from build123d import *

# Parameters (mm, degrees)
F1_DEPTH = 3


with BuildPart() as f1:
    # F0 (on Front) → F1 (new body)
    with BuildSketch(Plane.XZ):
        with BuildLine():
            Line((11.384419, 13.364318), (16.65998, 18.639879))
            ThreePointArc((16.65998, 18.639879), (9.567086, 23.096988), (1.4, 24.960769))
            Line((1.4, 24.960769), (1.4, 17.5))
            Line((1.4, 17.5), (-1.4, 17.5))
            Line((-1.4, 17.5), (-1.4, 24.960769))
            ThreePointArc((-1.4, 24.960769), (-9.567086, 23.096988), (-16.65998, 18.639879))
            Line((-16.65998, 18.639879), (-11.384419, 13.364318))
            Line((-11.384419, 13.364318), (-13.364318, 11.384419))
            Line((-13.364318, 11.384419), (-18.639879, 16.65998))
            ThreePointArc((-18.639879, 16.65998), (-23.096988, 9.567086), (-24.960769, 1.4))
            Line((-24.960769, 1.4), (-17.5, 1.4))
            Line((-17.5, 1.4), (-17.5, -1.4))
            Line((-17.5, -1.4), (-24.960769, -1.4))
            ThreePointArc((-24.960769, -1.4), (-23.096988, -9.567086), (-18.639879, -16.65998))
            Line((-18.639879, -16.65998), (-13.364318, -11.384419))
            Line((-13.364318, -11.384419), (-11.384419, -13.364318))
            Line((-11.384419, -13.364318), (-16.65998, -18.639879))
            ThreePointArc((-16.65998, -18.639879), (-9.567086, -23.096988), (-1.4, -24.960769))
            Line((-1.4, -24.960769), (-1.4, -17.5))
            Line((-1.4, -17.5), (1.4, -17.5))
            Line((1.4, -17.5), (1.4, -24.960769))
            ThreePointArc((1.4, -24.960769), (9.567086, -23.096988), (16.65998, -18.639879))
            Line((16.65998, -18.639879), (11.384419, -13.364318))
            Line((11.384419, -13.364318), (13.364318, -11.384419))
            Line((13.364318, -11.384419), (18.639879, -16.65998))
            ThreePointArc((18.639879, -16.65998), (23.096988, -9.567086), (24.960769, -1.4))
            Line((24.960769, -1.4), (17.5, -1.4))
            Line((17.5, -1.4), (17.5, 1.4))
            Line((17.5, 1.4), (24.960769, 1.4))
            ThreePointArc((24.960769, 1.4), (23.096988, 9.567086), (18.639879, 16.65998))
            Line((18.639879, 16.65998), (13.364318, 11.384419))
            Line((13.364318, 11.384419), (11.384419, 13.364318))
        make_face()
    extrude(amount=F1_DEPTH)


solid = f1.part
Geometry check sheet. Reference: the model listing, model coordinates, mm. A direction names the side the tool comes from. Give positions to 0.01 mm unless a question says otherwise; leave off trailing zeros. Order: outer loops, then holes, each group sorted by start corner. A loop starts at its lowest first (then second) coordinate and runs counter-clockwise, first axis right, second up. Notation, with made-up numbers: M 40.5,84.25 L 86.5,84.25 A20 ccw 86.5,116.25 Z; hole C -12,26.5 d3. An arc over 180 degrees is marked long. Use a Markdown table: item, result.
Item 1: Tool access check on faces 1 (the flat face through (-17.5, -1, 0)), 2 (the flat face through (-1.4, -1, -21)), 3 (the flat face through (-15.97, -1.48, 13.99)), 4 (the flat face through (21, -1, -1.4)). Record the directions out of +Z, -Z, +X, -X, +Y, -Y that give a thin tool (end or side, any length) a straight path to the whole face; none if there is none.
Answers follow:
| item | result |
|---|---|
| face 1 | -X, +Y, -Y |
| face 2 | -Z, +Y, -Y |
| face 3 | +Y, -Y |
| face 4 | +X, +Y, -Y |
Item 2: Draft check along X on faces 5 (the cylindrical face through (23.05, -1.48, -9.68)), 6 (the flat face through (0, -3, 0)), 7 (the flat face through (16.04, -1.48, 14.06)), 8 (the flat face through (14.06, -1.48, -16.04)). Enter one of: +X half, -X half, draft (parallel to the pull), parting line (faces both ways), or undercut.
Answers follow:
| item | result |
|---|---|
| face 5 | +X half |
| face 6 | draft |
| face 7 | undercut |
| face 8 | undercut |
Item 3: Section check B-B (x = -15). Record the cut outline in (y, z), and give its area (3 significant figures).
Answers follow:
| item | result |
|---|---|
| outline | M -3,-20 L 0,-20 L 0,-16.98 L -3,-16.98 Z; M -3,-13.02 L 0,-13.02 L 0,13.02 L -3,13.02 Z; M -3,16.98 L 0,16.98 L 0,20 L -3,20 Z |
| area | 96.2 mm2 |
Item 4: Material ranges on line 1 along X through (y, z) = (-1.25, 14); line 2 along Z through (x, y) = (-16, -1.7); line 3 along Z through (x, y) = (-15, -2.1), recorded low to high.
Answers follow:
| item | result |
|---|---|
| line 1 | x = -20.71 to -15.98, -12.02 to 12.02, 15.98 to 20.71 |
| line 2 | z = -19.21 to -17.98, -14.02 to 14.02, 17.98 to 19.21 |
| line 3 | z = -20 to -16.98, -13.02 to 13.02, 16.98 to 20 |
Item 5: Section check A-A (z = 15). Record the cut outline in (x, y), and give its area (3 significant figures).
Answers follow:
| item | result |
|---|---|
| outline | M -20,-3 L -16.98,-3 L -16.98,0 L -20,0 Z; M -13.02,-3 L 13.02,-3 L 13.02,0 L -13.02,0 Z; M 16.98,-3 L 20,-3 L 20,0 L 16.98,0 Z |
| area | 96.2 mm2 |
Item 6: Depth check by flat-ended pin: P1, Ø1.5, axis at y = -1, z = 20, coming from the +X side; P2, Ø1.4, axis at x = 0, y = -2, coming from the -Z side; P3, Ø0.8, axis at y = -2, z = -0.5, coming from the +X side. Enter the tip coordinate at first touch or a pass-through.
Answers follow:
| item | result |
|---|---|
| P1 | stops at x = 15.95 |
| P2 | stops at z = -17.5 |
| P3 | stops at x = 17.5 |
Item 7: Section check D-D (x = 20.5). Record the cut outline in (y, z).
Answers follow:
| item | result |
|---|---|
| outline | M -3,-14.31 L 0,-14.31 L 0,-1.4 L -3,-1.4 Z; M -3,1.4 L 0,1.4 L 0,14.31 L -3,14.31 Z |
